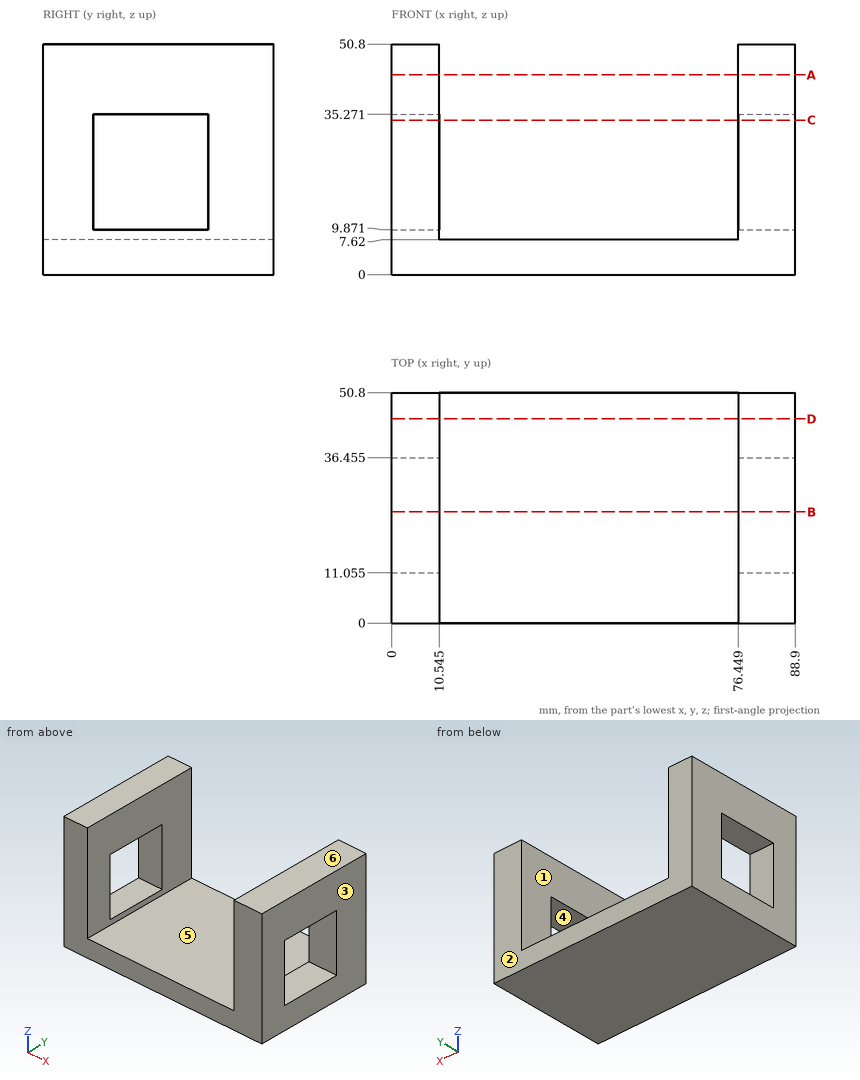
Print and shaded views of the part. All mm, measured from the part's lowest x, y and z. A direction names the side the tool comes from. Round coordinates to 2 decimals unless told otherwise and drop trailing zeros. Order: outer loops, then holes, each group sorted by start corner. A loop starts at its lowest first (then second) coordinate and runs counter-clockwise, first axis right, second up. Notation, with made-up numbers: (-30, 4.25) - (15, 4.25) arc R23 ccw to (15, 15.25) - close; hole circle Ø3 at (-11, 39). An arc over 180 degrees is marked (long way). Use a Markdown table: item, result.
1) Saw through at D-D on y = 45. Write the cut outline in (x, z) (1 decimal), and give its area (3 significant figures).
Recorded:
| item | result |
|---|---|
| outline | (0, 0) - (88.9, 0) - (88.9, 50.8) - (76.4, 50.8) - (76.4, 7.6) - (10.5, 7.6) - (10.5, 50.8) - (0, 50.8) - close |
| area | 1,670 mm² |
2) Wall check: L1, parallel to X at y = 13, z = 42.5 (1 decimal); L2, parallel to Y at x = 80, z = 29.5 (1 decimal); L3, parallel to Z at x = 76.5, y = 25. Give the ranges that are in metal, low to high.
Recorded:
| item | result |
|---|---|
| L1 | x = 0 to 10.5, 76.4 to 88.9 |
| L2 | y = 0 to 11.1, 36.5 to 50.8 |
| L3 | z = 0 to 9.87, 35.27 to 50.8 |
3) Saw through at C-C on z = 34. Write the cut outline in (x, y) (1 decimal), and give its area (3 significant figures).
Recorded:
| item | result |
|---|---|
| outline | (0, 0) - (10.5, 0) - (10.5, 11.1) - (0, 11.1) - close; (0, 36.5) - (10.5, 36.5) - (10.5, 50.8) - (0, 50.8) - close; (76.4, 0) - (88.9, 0) - (88.9, 11.1) - (76.4, 11.1) - close; (76.4, 36.5) - (88.9, 36.5) - (88.9, 50.8) - (76.4, 50.8) - close |
| area | 584 mm² |
4) Saw through at B-B on y = 24.5. Write the cut outline in (x, z) (1 decimal), and give its area (3 significant figures).
Recorded:
| item | result |
|---|---|
| outline | (0, 0) - (88.9, 0) - (88.9, 9.9) - (76.4, 9.9) - (76.4, 7.6) - (10.5, 7.6) - (10.5, 9.9) - (0, 9.9) - close; (0, 35.3) - (10.5, 35.3) - (10.5, 50.8) - (0, 50.8) - close; (76.4, 35.3) - (88.9, 35.3) - (88.9, 50.8) - (76.4, 50.8) - close |
| area | 1,090 mm² |
5) Flat gauge pins, fed straight in: pin 1 Ø10 at (x, y) = (48, 32) entering from +Z; pin 2 Ø10 at (x, z) = (69.5, 14) entering from +Y. Where does each tip first touch, or does it go through?
Recorded:
| item | result |
|---|---|
| pin 1 | stops at z = 7.62 |
| pin 2 | passes through |
6) Pull direction X, two halves, no side cores. Call the marked faces 1, 2 and 3: pulls with the +X half, pulls with the -X half, needs draft (parallel to the pull), parting line crosses it, or undercut.
Recorded:
| item | result |
|---|---|
| face 1 | undercut |
| face 2 | needs draft |
| face 3 | pulls with the +X half |
7) Saw through at A-A on z = 44. Write the cut outline in (x, y) (1 decimal), and give its area (3 significant figures).
Recorded:
| item | result |
|---|---|
| outline | (0, 0) - (10.5, 0) - (10.5, 50.8) - (0, 50.8) - close; (76.4, 0) - (88.9, 0) - (88.9, 50.8) - (76.4, 50.8) - close |
| area | 1,170 mm² |
8) Tool access for the marked faces 4, 5 and 6: list every direction of +Z, -Z, +X, -X, +Y, -Y with a clear straight run to the whole face (end or side of a thin tool).
Recorded:
| item | result |
|---|---|
| face 4 | +X, -X |
| face 5 | +Z, +Y, -Y |
| face 6 | +Z, +X, -X, +Y, -Y |
